```python
from build123d import *

# Parameters (mm, degrees)
SKETCH1_W          = 0.01
SKETCH1_H          = 4
SKETCH1_W_2        = 2
SKETCH1_H_2        = 20
CUT_EXTRUDE1_REACH = 32
SKETCH2_R          = 0.6
CHAMFER1_SIZE      = 0.5


with BuildPart() as part:
    # Sketch1 → Revolve1 (revolve)
    with BuildSketch(Plane.XY, mode=Mode.PRIVATE) as revolve1_sk:
        with BuildLine():
            Line((0, 14.630942634), (0, 13.230942634))
            ThreePointArc((0, 13.230942634), (5.719297581, 10.578866966), (7.39, 4.5))
            Line((7.39, 4.5), (7.99, 4.5))
            Line((7.99, 4.5), (7.99, 8.5))
            ThreePointArc((7.99, 8.5), (5.035587294, 12.921591081), (0, 14.630942634))
        make_face()
        with Locations((7.995, 6.5)):
            Rectangle(SKETCH1_W, SKETCH1_H)
        with Locations((9, 10)):
            Rectangle(SKETCH1_W_2, SKETCH1_H_2)
    revolve(revolve1_sk.sketch.rotate(Axis((0, 0, 0), (0, 1, 0)), 90), axis=Axis((0, 0, 0), (0, 1, 0)))

    # Sketch2 → Cut-Extrude1 (cut, up to next)
    with BuildSketch(Plane(origin=(10, 0, 0), x_dir=(0, 0, -1), z_dir=(1, 0, 0)), mode=Mode.PRIVATE) as cut_extrude1_sk1:
        with Locations((0, 16)):
            Circle(SKETCH2_R)
    cut_extrude1_tool1 = extrude(cut_extrude1_sk1.sketch, amount=-CUT_EXTRUDE1_REACH, mode=Mode.PRIVATE) & part.part
    # Sketch2 → Cut-Extrude1 (cut, up to next)
    with BuildSketch(Plane(origin=(10, 0, 0), x_dir=(0, 0, -1), z_dir=(1, 0, 0)), mode=Mode.PRIVATE) as cut_extrude1_sk2:
        with Locations((0, 4)):
            Circle(SKETCH2_R)
    cut_extrude1_tool2 = extrude(cut_extrude1_sk2.sketch, amount=-CUT_EXTRUDE1_REACH, mode=Mode.PRIVATE) & part.part
    add(cut_extrude1_tool1.solids().sort_by_distance((10, 16, 0))[0], mode=Mode.SUBTRACT)
    add(cut_extrude1_tool2.solids().sort_by_distance((10, 4, 0))[0], mode=Mode.SUBTRACT)

    # Chamfer1
    # the kernel refuses this chamfer: 1, 0.5 mm, written as the material it takes off along each edge
    with BuildSketch(Plane(origin=(0, 4.5, 0), x_dir=(0, 0, -1), z_dir=(1, 0, 0))) as chamfer1_piece_1:
        with BuildLine():
            Line((7.39 + CHAMFER1_SIZE, 0), (7.492670793, 1.1705165))
            ThreePointArc((7.492670793, 1.1705165), (7.465898714, 0.601555049), (7.39, 0))
            Line((7.39, 0), (7.39 + CHAMFER1_SIZE, 0))
        make_face()
    revolve(axis=Axis((0, 4.5, 0), (0, 1, 0)), revolution_arc=290.997944541, mode=Mode.SUBTRACT)
    with BuildSketch(Plane(origin=(0, 4.5, 0), x_dir=(0.9340589469331272, 0, 0.3571188648813968), z_dir=(-0.3571188648813968, 0, 0.9340589469331272))) as chamfer1_piece_2:
        with BuildLine():
            Line((7.39 + CHAMFER1_SIZE, 0), (7.492670793, 1.1705165))
            ThreePointArc((7.492670793, 1.1705165), (7.465898714, 0.601555049), (7.39, 0))
            Line((7.39, 0), (7.39 + CHAMFER1_SIZE, 0))
        make_face()
    revolve(axis=Axis((0, 4.5, 0), (0, 1, 0)), revolution_arc=110.92336072, mode=Mode.SUBTRACT)


solid = part.part
```
Input: part model. Units: mm. Frame: model coordinates. A direction names the side the tool comes from. Give positions to 0.01 mm unless a question says otherwise; leave off trailing zeros. Write each loop counter-clockwise with the first axis right and the second up, starting at its lowest first coordinate (ties: lowest second). Pieces come first, ordered by that corner, then holes. Notation, with made-up numbers: (58.5, 67.25) - (86.5, 67.25) arc R22 cw to (86.5, 104.25) - close; hole circle Ø1 at (40, -8.75). An arc over 180 degrees is marked (long way). Write item = value, one per line. Start each with the question number.
1) Material intervals for L1, parallel to Y at x = 8.6, z = 0; L2, parallel to X at y = 9.75, z = -2.5; L3, parallel to X at y = 13.75, z = 0, sorted ascending. Write a range as [from, to].
2) Pin query (flat end, axial travel): pin 1 (2 mm diameter, centred on x = 4.5, y = 7, fed in from -Z); pin 2 (6 mm diameter, centred on y = 3, z = 8, fed in from -X); pin 3 (3 mm diameter, centred on y = 15, z = 8, fed in from -X). Return the tip coordinate at first contact, or that it passes through.
3) Reachability of faces 1 (the face through (7.81, 14.33, 1.73)), 2 (the face through (-8.2, 0, 0)), 3 (the face through (9.003, 16.595, 0.078)) from +Z, -Z, +X, -X, +Y, -Y: full face, straight path, thin tool, end or side. Return the list, or none.
4) Cut plane A-A (y = 12.5). Return loops of the section in (x, z), and give its area (3 significant figures).
5) Draft query along Z for faces 4 (the face through (-8.2, 20, 0)), 5 (the face through (8.943, 4.595, 0.078)), 6 (the face through (0, 10, 10)), 7 (the face through (7.81, 2.28, 1.73)). Return one class per face: pulls with the +Z half, pulls with the -Z half, needs draft (parallel to the pull), parting line crosses it, or undercut.
6) Cut plane D-D (y = 2.25). Return loops of the section in (x, z), and give its area (3 significant figures).
7) Cut plane B-B (z = 0). Give the number of separate pieces and of enclosed holes in the cut face, and give its area (3 significant figures).
Answers follow:
q1.L1 = [0, 3.4], [4.6, 15.4], [16.6, 20]
q1.L2 = [-9.68, -7.6], [-7.12, -5.81], [5.81, 7.12], [7.6, 9.68]
q1.L3 = [-10, -8], [-3.71, 3.71], [8, 10]
q2.pin_1 = -9.37
q2.pin_2 = -8.66
q2.pin_3 = -7.6
q3.face_1 = +Y
q3.face_2 = +Z, -Z, +X, -X, -Y
q3.face_3 = +X
q4.outline = circle Ø20 at (0, 0); circle Ø11.08 at (0, 0); hole circle Ø16 at (0, 0); hole circle Ø6.46 at (0, 0)
q4.area = 177 mm^2
q5.face_4 = needs draft
q5.face_5 = undercut
q5.face_6 = parting line crosses it
q5.face_7 = undercut
q6.outline = circle Ø20 at (0, 0); hole circle Ø16 at (0, 0)
q6.area = 113 mm^2
q7.separate_pieces = 3
q7.enclosed_holes = 0
q7.area = 104 mm^2
